from build123d import *

# Parameters (mm, degrees)
SKETCH1_W                    = 45
SKETCH1_H                    = 45
SKETCH1_R                    = 15.5
SKETCH1_R_2                  = 1.5
BASE_FLANGE1_DEPTH           = 2
EDGE_FLANGE1_STRIP_W         = 14
EDGE_FLANGE1_STRIP_H         = 2
EDGE_FLANGE1_STRIP_CUT_DEPTH = 45
EDGE_FLANGE1_DEPTH           = 45
EDGE_FLANGE2_STRIP_W         = 14
EDGE_FLANGE2_STRIP_H         = 2
EDGE_FLANGE2_STRIP_CUT_DEPTH = 45
EDGE_FLANGE2_DEPTH           = 45
EDGE_FLANGE3_STRIP_W         = 14
EDGE_FLANGE3_STRIP_H         = 2
EDGE_FLANGE3_STRIP_CUT_DEPTH = 45
EDGE_FLANGE3_DEPTH           = 45
EDGE_FLANGE4_STRIP_W         = 14
EDGE_FLANGE4_STRIP_H         = 2
EDGE_FLANGE4_STRIP_CUT_DEPTH = 45
EDGE_FLANGE4_DEPTH           = 45
SKETCH18_R                   = 1.5
CUT_EXTRUDE1_DEPTH           = 10
SKETCH19_R                   = 1.5
CUT_EXTRUDE2_DEPTH           = 10


# Sheet-metal steps are written as plain solids
with BuildPart() as part:
    # Sketch1 → Base-Flange1 (new body)
    with BuildSketch(Plane.XY):
        Rectangle(SKETCH1_W, SKETCH1_H)
        Circle(SKETCH1_R, mode=Mode.SUBTRACT)
        with Locations((-15.5, 15.5)):
            Circle(SKETCH1_R_2, mode=Mode.SUBTRACT)
        with Locations((15.5, 15.5)):
            Circle(SKETCH1_R_2, mode=Mode.SUBTRACT)
        with Locations((15.5, -15.5)):
            Circle(SKETCH1_R_2, mode=Mode.SUBTRACT)
        with Locations((-15.5, -15.5)):
            Circle(SKETCH1_R_2, mode=Mode.SUBTRACT)
    extrude(amount=-BASE_FLANGE1_DEPTH)

    # Edge-Flange1 strip (across the edge) → Edge-Flange1 strip cut (cut)
    with BuildSketch(Plane(origin=(22.5, 22.5, -2), x_dir=(-1, 0, 0), z_dir=(0, -1, 0))):
        with Locations((-2, -1)):
            Rectangle(EDGE_FLANGE1_STRIP_W, EDGE_FLANGE1_STRIP_H)
    extrude(amount=EDGE_FLANGE1_STRIP_CUT_DEPTH, mode=Mode.SUBTRACT)

    # Edge-Flange1 section (across the edge) → Edge-Flange1 (add)
    with BuildSketch(Plane(origin=(22.5, 22.5, -2), x_dir=(-1, 0, 0), z_dir=(0, -1, 0))):
        with BuildLine():
            Line((0, 3), (0, 25.5))
            Line((0, 25.5), (2, 25.5))
            Line((2, 25.5), (2, 3))
            ThreePointArc((2, 3), (2.878679656, 0.878679656), (5, 0))
            Line((5, 0), (5, -2))
            ThreePointArc((5, -2), (1.464466094, -0.535533906), (0, 3))
        make_face()
    extrude(amount=EDGE_FLANGE1_DEPTH)

    # Edge-Flange2 strip (across the edge) → Edge-Flange2 strip cut (cut)
    with BuildSketch(Plane(origin=(22.5, -22.5, -27.5), x_dir=(0, 0, 1), z_dir=(0, 1, 0))):
        with Locations((-2, -1)):
            Rectangle(EDGE_FLANGE2_STRIP_W, EDGE_FLANGE2_STRIP_H)
    extrude(amount=EDGE_FLANGE2_STRIP_CUT_DEPTH, mode=Mode.SUBTRACT)

    # Edge-Flange2 section (across the edge) → Edge-Flange2 (add)
    with BuildSketch(Plane(origin=(22.5, -22.5, -27.5), x_dir=(0, 0, 1), z_dir=(0, 1, 0))):
        with BuildLine():
            Line((0, 3), (0, 18))
            Line((0, 18), (2, 18))
            Line((2, 18), (2, 3))
            ThreePointArc((2, 3), (2.878679656, 0.878679656), (5, 0))
            Line((5, 0), (5, -2))
            ThreePointArc((5, -2), (1.464466094, -0.535533906), (0, 3))
        make_face()
    extrude(amount=EDGE_FLANGE2_DEPTH)

    # Edge-Flange3 strip (across the edge) → Edge-Flange3 strip cut (cut)
    with BuildSketch(Plane(origin=(-22.5, -22.5, -2), x_dir=(1, 0, 0), z_dir=(0, 1, 0))):
        with Locations((-2, -1)):
            Rectangle(EDGE_FLANGE3_STRIP_W, EDGE_FLANGE3_STRIP_H)
    extrude(amount=EDGE_FLANGE3_STRIP_CUT_DEPTH, mode=Mode.SUBTRACT)

    # Edge-Flange3 section (across the edge) → Edge-Flange3 (add)
    with BuildSketch(Plane(origin=(-22.5, -22.5, -2), x_dir=(1, 0, 0), z_dir=(0, 1, 0))):
        with BuildLine():
            Line((0, 3), (0, 25.5))
            Line((0, 25.5), (2, 25.5))
            Line((2, 25.5), (2, 3))
            ThreePointArc((2, 3), (2.878679656, 0.878679656), (5, 0))
            Line((5, 0), (5, -2))
            ThreePointArc((5, -2), (1.464466094, -0.535533906), (0, 3))
        make_face()
    extrude(amount=EDGE_FLANGE3_DEPTH)

    # Edge-Flange4 strip (across the edge) → Edge-Flange4 strip cut (cut)
    with BuildSketch(Plane(origin=(-22.5, 22.5, -27.5), x_dir=(0, 0, 1), z_dir=(0, -1, 0))):
        with Locations((-2, -1)):
            Rectangle(EDGE_FLANGE4_STRIP_W, EDGE_FLANGE4_STRIP_H)
    extrude(amount=EDGE_FLANGE4_STRIP_CUT_DEPTH, mode=Mode.SUBTRACT)

    # Edge-Flange4 section (across the edge) → Edge-Flange4 (add)
    with BuildSketch(Plane(origin=(-22.5, 22.5, -27.5), x_dir=(0, 0, 1), z_dir=(0, -1, 0))):
        with BuildLine():
            Line((0, 3), (0, 18))
            Line((0, 18), (2, 18))
            Line((2, 18), (2, 3))
            ThreePointArc((2, 3), (2.878679656, 0.878679656), (5, 0))
            Line((5, 0), (5, -2))
            ThreePointArc((5, -2), (1.464466094, -0.535533906), (0, 3))
        make_face()
    extrude(amount=EDGE_FLANGE4_DEPTH)

    # Sketch18 → Cut-Extrude1 (cut)
    with BuildSketch(Plane.XY.offset(-25.5)):
        with Locations((-33, 12.5)):
            Circle(SKETCH18_R)
        with Locations((-33, -12.5)):
            Circle(SKETCH18_R)
    extrude(amount=-CUT_EXTRUDE1_DEPTH, mode=Mode.SUBTRACT)

    # Sketch19 → Cut-Extrude2 (cut)
    with BuildSketch(Plane.XY.offset(-25.5)):
        with Locations((33, 12.5)):
            Circle(SKETCH19_R)
        with Locations((33, -12.5)):
            Circle(SKETCH19_R)
    extrude(amount=-CUT_EXTRUDE2_DEPTH, mode=Mode.SUBTRACT)


solid = part.part
Here's how the part is built. I have some questions about the finished solid (model axes, mm). A direction names the side the tool comes from. Round coordinates to 2 decimals unless told otherwise and drop trailing zeros. Write each loop counter-clockwise with the first axis right and the second up, starting at its lowest first coordinate (ties: lowest second). Pieces come first, ordered by that corner, then holes.
1. Suppose I cut it at B-B (z = -11.25). List the corners of the cut face in (x, y) for me.
2. Suppose I cut it at D-D (y = 12.5). State how many separate pieces and enclosed holes the cut face has, and give its area (3 significant figures).
3. Suppose I cut it at C-C (y = -9). List the corners of the cut face in (x, z) for me.
4. For faces 1 (the flat face through (-33, 0, -25.5)), 2 (the cylindrical face through (-19.64, -0.32, -2.9)), 3 (the flat face through (22.5, 0, -14)), which set-ups out of +Z, -Z, +X, -X, +Y, -Y let a thin tool reach every point of the face, with its end or its side?
5. I need wall thicknesses on L1, parallel to Y at x = -33, z = -26.7; L2, parallel to X at y = 16.5, z = -5.75; L3, parallel to Y at x = 0, z = -1.2. Which ranges of each line are inside material? Lowest first, please.
6. Suppose I cut it at A-A (x = 33). List the corners of the cut face in (y, z) for me, and give its area (3 significant figures).
7. Will these pins go through, and if not, where does the flat tip stop? pin 1 Ø17.5 at (x, y) = (4.5, -1) entering from -Z; pin 2 Ø4 at (x, y) = (-15.5, 15.5) entering from +Z; pin 3 Ø1 at (y, z) = (4, -5.5) entering from +X; pin 4 Ø1 at (y, z) = (-7, -17) entering from -X.
Answer sheet:
1. outline: (-22.5, -22.5) - (-20.5, -22.5) - (-20.5, 22.5) - (-22.5, 22.5) - close; (20.5, -22.5) - (22.5, -22.5) - (22.5, 22.5) - (20.5, 22.5) - close
2. separate pieces: 4
2. enclosed holes: 0
2. area: 202 mm2
3. outline: (-40.5, -27.5) - (-25.5, -27.5) arc R5 ccw to (-20.5, -22.5) - (-20.5, -5) arc R3 cw to (-17.5, -2) - (-12.62, -2) - (-12.62, 0) - (-17.5, 0) arc R5 ccw to (-22.5, -5) - (-22.5, -22.5) arc R3 cw to (-25.5, -25.5) - (-40.5, -25.5) - close; (12.62, -2) - (17.5, -2) arc R3 cw to (20.5, -5) - (20.5, -22.5) arc R5 ccw to (25.5, -27.5) - (40.5, -27.5) - (40.5, -25.5) - (25.5, -25.5) arc R3 cw to (22.5, -22.5) - (22.5, -5) arc R5 ccw to (17.5, 0) - (12.62, 0) - close
4. face 1: +Z, -X, +Y, -Y
4. face 2: -Z, +Y, -Y
4. face 3: +Z, +X, +Y, -Y
5. L1: y = -22.5 to -14, -11 to 11, 14 to 22.5
5. L2: x = -22.5 to -20.5, 20.5 to 22.5
5. L3: y = -22.5 to -15.5, 15.5 to 22.5
6. outline: (-22.5, -27.5) - (-14, -27.5) - (-14, -25.5) - (-22.5, -25.5) - close; (-11, -27.5) - (11, -27.5) - (11, -25.5) - (-11, -25.5) - close; (14, -27.5) - (22.5, -27.5) - (22.5, -25.5) - (14, -25.5) - close
6. area: 78.0 mm2
7. pin 1: passes through
7. pin 2: stops at z = 0
7. pin 3: stops at x = 22.5
7. pin 4: stops at x = -22.5
